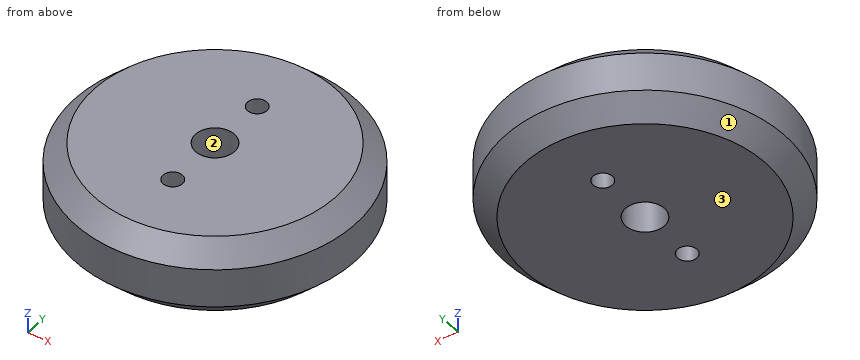
from build123d import *

# Parameters (mm, degrees)
SKETCH_1_R      = 36
SKETCH_1_R_2    = 5
SKETCH_1_R_3    = 2.5
EXTRUDE_1_DEPTH = 20
CHAMFER_1_SIZE  = 5


with BuildPart() as part:
    # 草圖1 → 填料-伸長1 (new body)
    with BuildSketch(Plane.XY):
        Circle(SKETCH_1_R)
        Circle(SKETCH_1_R_2, mode=Mode.SUBTRACT)
        with Locations((0, 15)):
            Circle(SKETCH_1_R_3, mode=Mode.SUBTRACT)
        with Locations((0, -15)):
            Circle(SKETCH_1_R_3, mode=Mode.SUBTRACT)
    extrude(amount=EXTRUDE_1_DEPTH)

    # 導角1
    chamfer_1_edges = [part.edges().sort_by_distance(p)[0] for p in [
        (-36, 0, 0),
        (-36, 0, 20),
    ]]
    chamfer(chamfer_1_edges, length=CHAMFER_1_SIZE)


solid = part.part
Geometry check sheet. Reference: the model listing, model coordinates, mm. Face numbers are marked on the shaded views. Round coordinates to 2 decimals unless told otherwise and drop trailing zeros. Write each loop counter-clockwise with the first axis right and the second up, starting at its lowest first coordinate (ties: lowest second). Pieces come first, ordered by that corner, then holes.
Item 1: Section check A-A (y = 0). Record the boundary of the cut face in (x, z).
Determined:
outline: (-36, 5) - (-31, 0) - (-5, 0) - (-5, 20) - (-31, 20) - (-36, 15) - close; (5, 0) - (31, 0) - (36, 5) - (36, 15) - (31, 20) - (5, 20) - close
Item 2: Section check C-C (z = 1.75). Record the boundary of the cut face in (x, y).
Determined:
outline: circle Ø65.5 at (0, 0); hole circle Ø10 at (0, 0); hole circle Ø5 at (0, -15); hole circle Ø5 at (0, 15)
Item 3: Material ranges on line 1 along Y through (x, z) = (0, 6.75); line 2 along X through (y, z) = (-0.5, 15.25); line 3 along Y through (x, z) = (-4.5, 12.5), recorded low to high.
Determined:
line 1: y = -36 to -17.5, -12.5 to -5, 5 to 12.5, 17.5 to 36
line 2: x = -35.75 to -4.97, 4.97 to 35.75
line 3: y = -35.72 to -2.18, 2.18 to 35.72
Item 4: Go/stop test with flat-tipped pins: pin 1 Ø10 at (x, y) = (28, -19.5) entering from -Z; pin 2 Ø2 at (x, z) = (-19.5, 7) entering from -Y; pin 3 Ø2 at (x, z) = (-14.5, 2) entering from -Y; pin 4 Ø6 at (x, z) = (-5.5, 3) entering from -Y. Record where each tip stops, or that it passes through.
Determined:
pin 1: stops at z = 0
pin 2: stops at y = -30.88
pin 3: stops at y = -30.85
pin 4: stops at y = -35.85
Item 5: Mould release check, pull along X, two halves, no side actions. Record for the marked faces 1, 2 and 3: +X half, -X half, draft (parallel to the pull), parting line (faces both ways), or undercut.
Determined:
face 1: parting line
face 2: undercut
face 3: draft
Item 6: Section check B-B (x = 0). Record the boundary of the cut face in (y, z), plus the area to 3 significant figures.
Determined:
outline: (-36, 5) - (-31, 0) - (-17.5, 0) - (-17.5, 20) - (-31, 20) - (-36, 15) - close; (-12.5, 0) - (-5, 0) - (-5, 20) - (-12.5, 20) - close; (5, 0) - (12.5, 0) - (12.5, 20) - (5, 20) - close; (17.5, 0) - (31, 0) - (36, 5) - (36, 15) - (31, 20) - (17.5, 20) - close
area: 990 mm2
Item 7: Section check D-D (z = 18.5). Record the boundary of the cut face in (x, y).
Determined:
outline: circle Ø65 at (0, 0); hole circle Ø10 at (0, 0); hole circle Ø5 at (0, -15); hole circle Ø5 at (0, 15)
